Read the model definition and answer for the solid it produces. Units are mm, in the model's axes. Round coordinates to 2 decimals unless told otherwise and drop trailing zeros. Order: outer loops, then holes, each group sorted by start corner. A loop starts at its lowest first (then second) coordinate and runs counter-clockwise, first axis right, second up. Notation, with made-up numbers: (77, -7) -> (97, -7) arc R25 ccw to (97, 15) -> close; hole circle Ø5 at (-23, 48.5). An arc over 180 degrees is marked (long way). One line per item, written item: value. Start each with the question number.
1. Section C-C (y = 58) is taken. Give the vertices of the cut face in (x, z) (3 decimals), then the cut area to 3 significant figures.
2. Section B-B (x = 14.5) is taken. Give the vertices of the cut face in (y, z) (3 decimals).
3. Flat-ended cylindrical pins translate along their axes: pin 1 Ø8 at (x, y) = (-11, 12.5) entering from +Z; pin 2 Ø0.8 at (x, z) = (-49, 0) entering from -Y. Find the tip coordinate at first contact, or state that the pin passes through.
4. Section A-A (y = 7) is taken. Give the vertices of the cut face in (x, z).
5. Consider line 1 (X direction, y = 0.5, z = 0); line 2 (X direction, y = -11, z = -0.2); line 3 (Y direction, x = 33, z = 0.4) (3 decimals). Determine where each line is inside the solid, lowest interval first.
6. Section D-D (z = 0.5) is taken. State how many separate pieces and enclosed holes the cut face has, then the cut area to 3 significant figures.
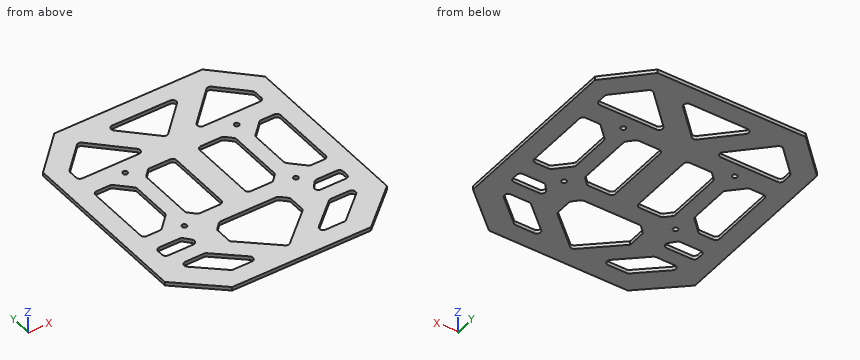
from build123d import *

# Parameters (mm, degrees)
BOSS_EXTRUDE1_DEPTH = 1.27
BOSS_EXTRUDE2_DEPTH = 2.54
SKETCH3_W           = 55.501519427
SKETCH3_H           = 49.578797493
CUT_EXTRUDE1_DEPTH  = 2.54
BOSS_EXTRUDE3_DEPTH = 2.54
BOSS_EXTRUDE4_DEPTH = 2.54
SKETCH6_R           = 1.65
CUT_EXTRUDE2_DEPTH  = 2.54
CHAMFER1_SIZE       = 5.08
FILLET1_R           = 2.54
FILLET2_R           = 2.54


with BuildPart() as part:
    # Sketch1 → Boss-Extrude1 (new, symmetric)
    with BuildSketch(Plane.XY):
        Polygon((-76.2, 60.325), (-76.2, -60.325), (76.2, -60.325), (76.2, 60.325), (50.8, 85.725), (-50.8, 85.725), align=None)
    extrude(amount=BOSS_EXTRUDE1_DEPTH, both=True)

    # Sketch2 → Boss-Extrude2 (add)
    with BuildSketch(Plane.XY.offset(1.27)):
        Polygon((-47.625, -85.725), (47.625, -85.725), (76.2, -60.325), (-76.2, -60.325), align=None)
    extrude(amount=-BOSS_EXTRUDE2_DEPTH)

    # Sketch3 → Cut-Extrude1 (cut)
    with BuildSketch(Plane.XY.offset(1.27)):
        Polygon((-25.107219952, -50.848797493), (-25.107219952, -33.068797493), (25.107219952, -33.068797493), (25.107219952, -50.848797493), (0, -73.166326339), align=None)
        Polygon((-62.895047936, -51.78188729), (-42.575047936, -51.78188729), (-18.676546137, -73.025), (-38.996546137, -73.025), align=None)
        Polygon((-25.913038854, 73.025), (25.913038854, 73.025), (0, 47.111961146), align=None)
        Polygon((18.676546137, -73.025), (38.996546137, -73.025), (62.895047936, -51.78188729), (42.575047936, -51.78188729), align=None)
        Polygon((-44.45, 71.755), (-63.5, 52.705), (-63.5, 43.301961146), (-15.996961146, 43.301961146), align=None)
        Polygon((44.45, 71.755), (63.5, 52.705), (63.5, 43.301961146), (15.996961146, 43.301961146), align=None)
        with Locations((-35.749240287, 4.420601253)):
            Rectangle(SKETCH3_W, SKETCH3_H)
        with Locations((35.749240287, 4.420601253)):
            Rectangle(SKETCH3_W, SKETCH3_H)
    extrude(amount=-CUT_EXTRUDE1_DEPTH, mode=Mode.SUBTRACT)

    # Sketch4 → Boss-Extrude3 (add)
    with BuildSketch(Plane.XY.offset(1.27)):
        Polygon((40.826553226, 29.21), (30.666553226, 29.21), (30.666553226, 24.01714149), (30.666553226, -15.175938983), (30.666553226, -20.368797493), (40.826553226, -20.368797493), (40.826553226, -12.82106127), (40.826553226, 21.662263777), align=None)
        Polygon((30.666553226, 24.01714149), (30.666553226, 29.21), (25.586553226, 29.21), align=None)
        Polygon((48.374289449, 29.21), (40.826553226, 29.21), (40.826553226, 21.662263777), align=None)
        Polygon((30.666553226, -20.368797493), (30.666553226, -15.175938983), (25.586553226, -20.368797493), align=None)
        Polygon((48.374289449, -20.368797493), (40.826553226, -12.82106127), (40.826553226, -20.368797493), align=None)
        Polygon((-25.586553226, 29.21), (-30.666553226, 29.21), (-30.666553226, 24.01714149), align=None)
        Polygon((-30.666553226, 24.01714149), (-30.666553226, 29.21), (-40.826553226, 29.21), (-40.826553226, 21.662263777), (-40.826553226, -12.82106127), (-40.826553226, -20.368797493), (-30.666553226, -20.368797493), (-30.666553226, -15.175938983), align=None)
        Polygon((-40.826553226, 21.662263777), (-40.826553226, 29.21), (-48.374289449, 29.21), align=None)
        Polygon((-25.586553226, -20.368797493), (-30.666553226, -15.175938983), (-30.666553226, -20.368797493), align=None)
        Polygon((-40.826553226, -20.368797493), (-40.826553226, -12.82106127), (-48.374289449, -20.368797493), align=None)
    extrude(amount=-BOSS_EXTRUDE3_DEPTH)

    # Sketch5 → Boss-Extrude4 (add)
    with BuildSketch(Plane.XY.offset(1.27)):
        Polygon((-40.826553226, 21.662263777), (-40.826553226, 19.122263777), (-50.914289449, 29.21), (-48.374289449, 29.21), align=None)
        Polygon((-48.374289449, -20.368797493), (-50.914289449, -20.368797493), (-40.826553226, -10.28106127), (-40.826553226, -12.82106127), align=None)
        Polygon((48.374289449, -20.368797493), (40.826553226, -12.82106127), (40.826553226, -10.28106127), (50.914289449, -20.368797493), align=None)
        Polygon((48.374289449, 29.21), (50.914289449, 29.21), (40.826553226, 19.122263777), (40.826553226, 21.662263777), align=None)
    extrude(amount=-BOSS_EXTRUDE4_DEPTH)

    # Sketch6 → Cut-Extrude2 (cut)
    with BuildSketch(Plane.XY.offset(1.27)):
        with Locations((38.250421337, 33.717772659)):
            Circle(SKETCH6_R)
        with Locations(Location((38.250421337, -24.876570152, 0), (0, 0, 180))):
            Circle(SKETCH6_R)
        with Locations((-38.250421337, -24.876570152)):
            Circle(SKETCH6_R)
        with Locations(Location((-38.250421337, 33.717772659, 0), (0, 0, 180))):
            Circle(SKETCH6_R)
        Polygon((45.870421337, -41.62188729), (63.5, -41.62188729), (63.5, -32.73188729), (45.870421337, -32.73188729), (38.250421337, -41.62188729), align=None)
        Polygon((-63.5, -41.62188729), (-63.5, -32.73188729), (-45.870421337, -32.73188729), (-38.250421337, -41.62188729), (-45.870421337, -41.62188729), align=None)
    extrude(amount=-CUT_EXTRUDE2_DEPTH, mode=Mode.SUBTRACT)

    # Chamfer1
    chamfer1_edges = [part.edges().sort_by_distance(p)[0] for p in [
        (-25.107219952, -33.068797493, 0),
        (25.107219952, -33.068797493, 0),
    ]]
    chamfer(chamfer1_edges, length=CHAMFER1_SIZE)

    # Fillet1
    fillet1_edges = [part.edges().sort_by_distance(p)[0] for p in [
        (25.107219952, -50.848797493, 0),
        (0, -73.166326339, 0),
        (38.250421337, -41.62188729, 0),
        (45.870421337, -32.73188729, 0),
        (63.5, -32.73188729, 0),
        (63.5, -41.62188729, 0),
        (-63.5, -41.62188729, 0),
        (-63.5, -32.73188729, 0),
        (-45.870421337, -32.73188729, 0),
        (-38.250421337, -41.62188729, 0),
        (-20.027219952, -33.068797493, 0),
        (20.027219952, -33.068797493, 0),
        (25.107219952, -38.148797493, 0),
        (-25.107219952, -38.148797493, 0),
        (-38.996546137, -73.025, 0),
        (-62.895047936, -51.78188729, 0),
        (-42.575047936, -51.78188729, 0),
        (-18.676546137, -73.025, 0),
        (18.676546137, -73.025, 0),
        (42.575047936, -51.78188729, 0),
        (62.895047936, -51.78188729, 0),
        (38.996546137, -73.025, 0),
    ]]
    fillet(fillet1_edges, radius=FILLET1_R)

    # Fillet2
    fillet2_edges = [part.edges().sort_by_distance(p)[0] for p in [
        (-44.45, 71.755, 0),
        (-15.996961146, 43.301961146, 0),
        (-63.5, 43.301961146, 0),
        (-63.5, 52.705, 0),
        (15.996961146, 43.301961146, 0),
        (44.45, 71.755, 0),
        (63.5, 52.705, 0),
        (63.5, 43.301961146, 0),
        (7.998480573, 29.21, 0),
        (63.5, 29.21, 0),
        (63.5, -20.368797493, 0),
        (7.998480573, -20.368797493, 0),
        (25.586553226, 29.21, 0),
        (30.666553226, -15.175938983, 0),
        (30.666553226, 24.01714149, 0),
        (25.586553226, -20.368797493, 0),
        (-25.586553226, -20.368797493, 0),
        (-30.666553226, -15.175938983, 0),
        (-30.666553226, 24.01714149, 0),
        (-50.914289449, -20.368797493, 0),
        (-40.826553226, -10.28106127, 0),
        (50.914289449, 29.21, 0),
        (40.826553226, 19.122263777, 0),
        (50.914289449, -20.368797493, 0),
        (40.826553226, -10.28106127, 0),
        (-50.914289449, 29.21, 0),
        (-40.826553226, 19.122263777, 0),
        (-7.998480573, -20.368797493, 0),
        (-63.5, -20.368797493, 0),
        (-63.5, 29.21, 0),
        (-7.998480573, 29.21, 0),
        (25.913038854, 73.025, 0),
        (0, 47.111961146, 0),
        (-25.913038854, 73.025, 0),
    ]]
    fillet(fillet2_edges, radius=FILLET2_R)


solid = part.part
Answer:
1. outline: (-76.2, -1.27) -> (-58.205, -1.27) -> (-58.205, 1.27) -> (-76.2, 1.27) -> close; (-30.695, -1.27) -> (-10.888, -1.27) -> (-10.888, 1.27) -> (-30.695, 1.27) -> close; (10.888, -1.27) -> (30.695, -1.27) -> (30.695, 1.27) -> (10.888, 1.27) -> close; (58.205, -1.27) -> (76.2, -1.27) -> (76.2, 1.27) -> (58.205, 1.27) -> close
1. area: 192 mm^2
2. outline: (-85.725, -1.27) -> (-60.277, -1.27) -> (-60.277, 1.27) -> (-85.725, 1.27) -> close; (-33.069, -1.27) -> (-20.369, -1.27) -> (-20.369, 1.27) -> (-33.069, 1.27) -> close; (29.21, -1.27) -> (61.612, -1.27) -> (61.612, 1.27) -> (29.21, 1.27) -> close; (73.025, -1.27) -> (85.725, -1.27) -> (85.725, 1.27) -> (73.025, 1.27) -> close
3. pin 1: z = 1.27
3. pin 2: y = -84.86
4. outline: (-76.2, -1.27) -> (-63.5, -1.27) -> (-63.5, 1.27) -> (-76.2, 1.27) -> close; (-40.83, -1.27) -> (-30.67, -1.27) -> (-30.67, 1.27) -> (-40.83, 1.27) -> close; (-8, -1.27) -> (8, -1.27) -> (8, 1.27) -> (-8, 1.27) -> close; (30.67, -1.27) -> (40.83, -1.27) -> (40.83, 1.27) -> (30.67, 1.27) -> close; (63.5, -1.27) -> (76.2, -1.27) -> (76.2, 1.27) -> (63.5, 1.27) -> close
5. line 1: -76.2 to -63.5, -40.83 to -30.67, -8 to 8, 30.67 to 40.83, 63.5 to 76.2
5. line 2: -76.2 to -63.5, -41.55 to -30.67, -8 to 8, 30.67 to 41.55, 63.5 to 76.2
5. line 3: -85.725 to -73.025, -60.293 to 43.302, 60.305 to 85.725
6. separate pieces: 1
6. enclosed holes: 16
6. area: 15,700 mm^2
